Verification items for the finished model (mm, model axes). Coordinates: 2 decimals unless noted, no trailing zeros. Write each loop counter-clockwise with the first axis right and the second up, starting at its lowest first coordinate (ties: lowest second). Pieces come first, ordered by that corner, then holes. Notation, with made-up numbers: (-24.5, 76) -> (-2.5, 76) arc R18 cw to (-2.5, 107) -> close; hole circle Ø7 at (53.5, 11). An arc over 180 degrees is marked (long way). Write item = value, one per line. Start each with the question number.
(1) Material ranges on probe 1 along X at (y, z) = (2, -63.5); probe 2 along Z at (x, y) = (63.5, 1.3); probe 3 along Z at (x, y) = (64, 2.2), recorded low to high. Write a range as [from, to].
(2) Gauge pin test, flat end, axial feed: pin 1 Ø4.5 at (x, z) = (6.35, -63.5) entering from -Y. Record the tip position at first contact, or that the pin passes through.
(3) Section check A-A (y = 1.95). Record the cut outline in (x, z), plus the area to 3 significant figures.
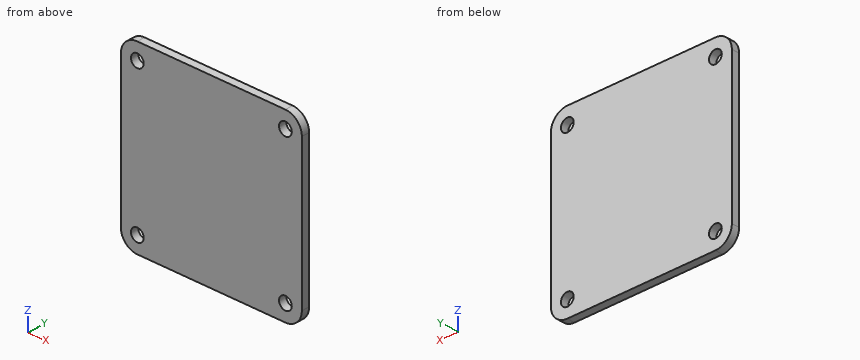
```python
from build123d import *

# Parameters (mm, degrees)
SKETCH1_W           = 69.85
SKETCH1_H           = 69.85
BOSS_EXTRUDE1_DEPTH = 3.048
SKETCH2_R           = 2.45999
CUT_EXTRUDE1_DEPTH  = 99.829830031
FILLET2_R           = 6.35


with BuildPart() as part:
    # Sketch1 → Boss-Extrude1 (new body)
    with BuildSketch(Plane(origin=(0, 0, 0), x_dir=(1, 0, 0), z_dir=(0, 1, 0))):
        with Locations((34.925, 34.925)):
            Rectangle(SKETCH1_W, SKETCH1_H)
    extrude(amount=BOSS_EXTRUDE1_DEPTH)

    # Sketch2 → Cut-Extrude1 (cut, through all)
    with BuildSketch(Plane(origin=(0, 0, 0), x_dir=(1, 0, 0), z_dir=(0, 1, 0))):
        with Locations(Location((6.35, 6.35, 0), (0, 0, 90))):
            Circle(SKETCH2_R)
        with Locations(Location((63.5, 6.35, 0), (0, 0, 90))):
            Circle(SKETCH2_R)
        with Locations(Location((6.35, 63.5, 0), (0, 0, 90))):
            Circle(SKETCH2_R)
        with Locations(Location((63.5, 63.5, 0), (0, 0, 90))):
            Circle(SKETCH2_R)
    extrude(amount=CUT_EXTRUDE1_DEPTH, mode=Mode.SUBTRACT)

    # Fillet2
    fillet2_edges = [part.edges().sort_by_distance(p)[0] for p in [
        (0, 1.524, -69.85),
        (69.85, 1.524, -69.85),
        (69.85, 1.524, 0),
        (0, 1.524, 0),
    ]]
    fillet(fillet2_edges, radius=FILLET2_R)


solid = part.part
```
Response:
q1.probe_1 = [0, 3.89], [8.81, 61.04], [65.96, 69.85]
q1.probe_2 = [-69.85, -65.96], [-61.04, -8.81], [-3.89, 0]
q1.probe_3 = [-69.83, -65.91], [-61.09, -8.76], [-3.94, -0.02]
q2.pin_1 = through
q3.outline = (0, -63.5) arc R6.35 ccw to (6.35, -69.85) -> (63.5, -69.85) arc R6.35 ccw to (69.85, -63.5) -> (69.85, -6.35) arc R6.35 ccw to (63.5, 0) -> (6.35, 0) arc R6.35 ccw to (0, -6.35) -> close; hole circle Ø4.92 at (6.35, -63.5); hole circle Ø4.92 at (6.35, -6.35); hole circle Ø4.92 at (63.5, -63.5); hole circle Ø4.92 at (63.5, -6.35)
q3.area = 4,770 mm2
